Job drawing, mm, ordinate dimensions from the low corner. One solid piece. A direction names the side the tool comes from. Give positions to 0.01 mm unless a question says otherwise; leave off trailing zeros. Order: outer loops, then holes, each group sorted by start corner. A loop starts at its lowest first (then second) coordinate and runs counter-clockwise, first axis right, second up.
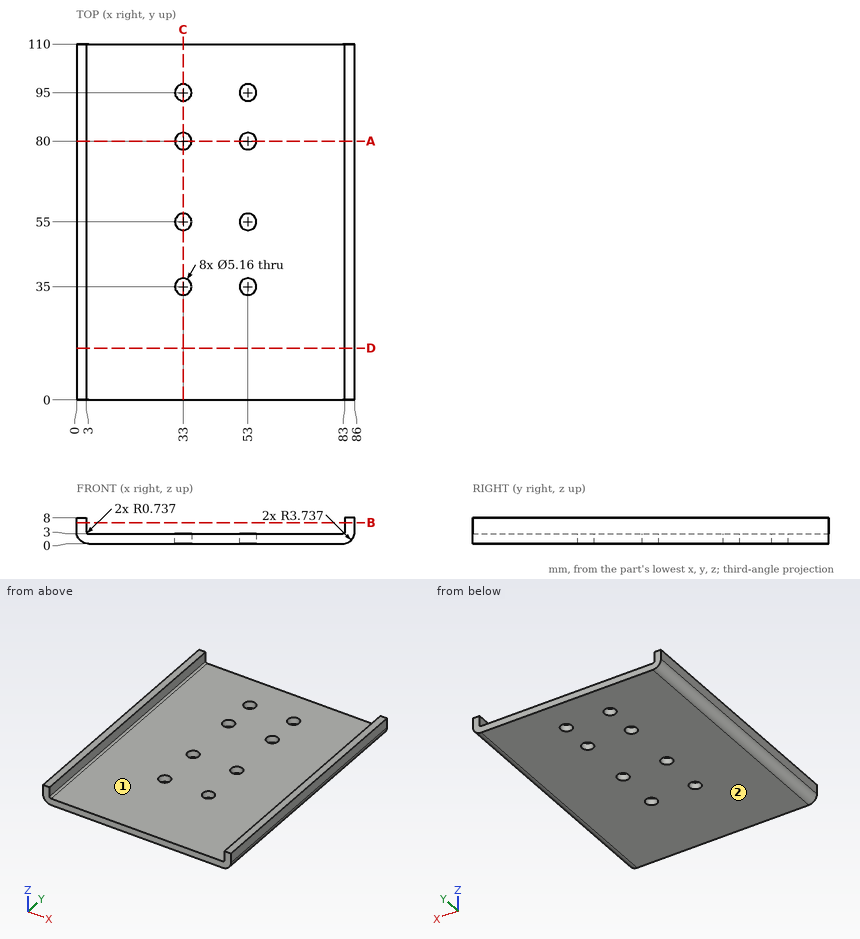
Item 1: Drop a flat-ended pin along its axis: P1, Ø2, axis at x = 14.5, y = 33, coming from the +Z side. Give the stop position or say it passes through.
Item 2: Band-saw the part on B-B on z = 6.5. List the corners of the cut face in (x, y), plus the area to 3 significant figures.
Item 3: Band-saw the part on A-A on y = 80. List the corners of the cut face in (x, z), plus the area to 3 significant figures.
Item 4: Band-saw the part on D-D on y = 16. List the corners of the cut face in (x, z), plus the area to 3 significant figures.
Item 5: Band-saw the part on C-C on x = 33. List the corners of the cut face in (y, z).
Item 6: Drill centre lines: probe 1 along Y at (x, z) = (53, 1.25); probe 2 along X at (y, z) = (59.5, 5); probe 3 along X at (y, z) = (95, 1.8). Where is each one in solid material? Low to high.
Item 7: Which spindle directions (+Z, -Z, +X, -X, +Y, -Y) get a long thin tool onto all of the face, cutting with end or side? Do the marked faces 1 and 2. Say none if no direction does.
Working result:
1. P1: stops at z = 3
2. outline: (0, 0) - (3, 0) - (3, 110) - (0, 110) - close; (83, 0) - (86, 0) - (86, 110) - (83, 110) - close
2. area: 660 mm2
3. outline: (0, 3.74) arc R3.74 ccw to (3.74, 0) - (30.42, 0) - (30.42, 3) - (3.74, 3) arc R0.74 cw to (3, 3.74) - (3, 8) - (0, 8) - close; (35.58, 0) - (50.42, 0) - (50.42, 3) - (35.58, 3) - close; (55.58, 0) - (82.26, 0) arc R3.74 ccw to (86, 3.74) - (86, 8) - (83, 8) - (83, 3.74) arc R0.74 cw to (82.26, 3) - (55.58, 3) - close
3. area: 251 mm2
4. outline: (0, 3.74) arc R3.74 ccw to (3.74, 0) - (82.26, 0) arc R3.74 ccw to (86, 3.74) - (86, 8) - (83, 8) - (83, 3.74) arc R0.74 cw to (82.26, 3) - (3.74, 3) arc R0.74 cw to (3, 3.74) - (3, 8) - (0, 8) - close
4. area: 282 mm2
5. outline: (0, 0) - (32.42, 0) - (32.42, 3) - (0, 3) - close; (37.58, 0) - (52.42, 0) - (52.42, 3) - (37.58, 3) - close; (57.58, 0) - (77.42, 0) - (77.42, 3) - (57.58, 3) - close; (82.58, 0) - (92.42, 0) - (92.42, 3) - (82.58, 3) - close; (97.58, 0) - (110, 0) - (110, 3) - (97.58, 3) - close
6. probe 1: y = 0 to 32.42, 37.58 to 52.42, 57.58 to 77.42, 82.58 to 92.42, 97.58 to 110
6. probe 2: x = 0 to 3, 83 to 86
6. probe 3: x = 0.54 to 30.42, 35.58 to 50.42, 55.58 to 85.46
7. face 1: +Z, +Y, -Y
7. face 2: -Z, +X, -X, +Y, -Y
